```python
from build123d import *

# Parameters (mm, degrees)
SKETCH1_R           = 22.5
SKETCH1_R_2         = 20
BOSS_EXTRUDE1_DEPTH = 3
SKETCH2_R           = 1.25
BOSS_EXTRUDE2_DEPTH = 3
CIRPATTERN1_COUNT   = 2
SKETCH3_R           = 6.6
BOSS_EXTRUDE3_DEPTH = 3
SKETCH4_R           = 2
CUT_EXTRUDE1_DEPTH  = 3


with BuildPart() as part:
    # Sketch1 → Boss-Extrude1 (new body)
    with BuildSketch(Plane(origin=(0, 0, 0), x_dir=(1, 0, 0), z_dir=(0, 1, 0))):
        with Locations(Location((0, 0, 0), (0, 0, 270))):
            Circle(SKETCH1_R)
        with Locations(Location((0, 0, 0), (0, 0, 270))):
            Circle(SKETCH1_R_2, mode=Mode.SUBTRACT)
    extrude(amount=BOSS_EXTRUDE1_DEPTH)

    # Sketch2 → Boss-Extrude2 (add)
    with BuildSketch(Plane(origin=(0, 0, 0), x_dir=(1, 0, 0), z_dir=(0, 1, 0))):
        with BuildLine():
            Line((-2.5, 27), (2.5, 27))
            Line((2.5, 27), (2.5, 22.360679775))
            ThreePointArc((2.5, 22.360679775), (0, 22.5), (-2.5, 22.360679775))
            Line((-2.5, 22.360679775), (-2.5, 27))
        make_face()
        with Locations(Location((0, 24.7, 0), (0, 0, 270))):
            Circle(SKETCH2_R, mode=Mode.SUBTRACT)
    boss_extrude2 = extrude(amount=BOSS_EXTRUDE2_DEPTH)

    # CirPattern1: Boss-Extrude2 ×2 about axis
    cirpattern1_axis = Axis((0, 0, 0), (0, 1, 0))
    for i in range(1, CIRPATTERN1_COUNT):
        add(boss_extrude2.rotate(cirpattern1_axis, i * 360 / CIRPATTERN1_COUNT))

    # Sketch3 → Boss-Extrude3 (add)
    with BuildSketch(Plane(origin=(0, 0, 0), x_dir=(1, 0, 0), z_dir=(0, 1, 0))):
        with BuildLine():
            Line((-3, 19.773719933), (-3, 7.95298686))
            ThreePointArc((-3, 7.95298686), (-6.535301084, 5.435056554), (-8.366600265, 1.5))
            Line((-8.366600265, 1.5), (-19.943670675, 1.5))
            ThreePointArc((-19.943670675, 1.5), (-20, 0), (-19.943670675, -1.5))
            Line((-19.943670675, -1.5), (-8.366600265, -1.5))
            ThreePointArc((-8.366600265, -1.5), (-6.535301084, -5.435056554), (-3, -7.95298686))
            Line((-3, -7.95298686), (-3, -19.773719933))
            ThreePointArc((-3, -19.773719933), (0, -20), (3, -19.773719933))
            Line((3, -19.773719933), (3, -7.95298686))
            ThreePointArc((3, -7.95298686), (6.535301084, -5.435056554), (8.366600265, -1.5))
            Line((8.366600265, -1.5), (19.943670675, -1.5))
            ThreePointArc((19.943670675, -1.5), (20, 0), (19.943670675, 1.5))
            Line((19.943670675, 1.5), (8.366600265, 1.5))
            ThreePointArc((8.366600265, 1.5), (6.535301084, 5.435056554), (3, 7.95298686))
            Line((3, 7.95298686), (3, 19.773719933))
            ThreePointArc((3, 19.773719933), (0, 20), (-3, 19.773719933))
        make_face()
        with Locations(Location((0, 0, 0), (0, 0, 270))):
            Circle(SKETCH3_R, mode=Mode.SUBTRACT)
    extrude(amount=BOSS_EXTRUDE3_DEPTH)

    # Sketch4 → Cut-Extrude1 (cut)
    with BuildSketch(Plane(origin=(0, 3, 0), x_dir=(1, 0, 0), z_dir=(0, 1, 0))):
        with Locations(Location((0, 12.5, 0), (0, 0, 270))):
            Circle(SKETCH4_R)
        with Locations(Location((0, -12.5, 0), (0, 0, 270))):
            Circle(SKETCH4_R)
    extrude(amount=-CUT_EXTRUDE1_DEPTH, mode=Mode.SUBTRACT)


solid = part.part
```
Can you work these out from the model? Positions are in its coordinate system, mm. A direction names the side the tool comes from. Coordinates: 2 decimals unless noted, no trailing zeros. Order: outer loops, then holes, each group sorted by start corner. A loop starts at its lowest first (then second) coordinate and runs counter-clockwise, first axis right, second up. Notation, with made-up numbers: (35, 35.5) - (43, 35.5) arc R15 cw to (43, 60.5) - close; hole circle Ø2 at (20, -8). An arc over 180 degrees is marked (long way). Answer in a Markdown table with one row per item.
1. If we mould it in two halves opening along Z, with no side actions, what happens to faces 5 (the cylindrical face through (-14.537, 1.479, -13.736)), 6 (the flat face through (-3.4, 0, 5.9)), 7 (the flat face through (0, 1, 27)), 8 (the flat face through (-3, 1, 14))? For each: pulls with the +Z half, pulls with the -Z half, needs draft (parallel to the pull), parting line crosses it, or undercut.
Reply:
| item | result |
|---|---|
| face 5 | undercut |
| face 6 | needs draft |
| face 7 | pulls with the +Z half |
| face 8 | undercut |
2. Suppose I cut it at A-A (z = -24.7). Please give me the cut outline in (x, y).
Reply:
| item | result |
|---|---|
| outline | (-2.5, 0) - (-1.25, 0) - (-1.25, 3) - (-2.5, 3) - close; (1.25, 0) - (2.5, 0) - (2.5, 3) - (1.25, 3) - close |
3. For faces 1 (the flat face through (-2.5, 1, -25)), 2 (the flat face through (2.5, 1, -25)), 3 (the flat face through (-2.5, 1, 25)), 4 (the cylindrical face through (6.5, 1.48, 5.48)), which set-ups out of +Z, -Z, +X, -X, +Y, -Y let a thin tool reach every point of the face, with its end or its side?
Reply:
| item | result |
|---|---|
| face 1 | -Z, -X, +Y, -Y |
| face 2 | -Z, +X, +Y, -Y |
| face 3 | +Z, -X, +Y, -Y |
| face 4 | +Y, -Y |
4. If I drill on line 1 along X through (y, z) = (1, -17); line 2 along Z through (x, y) = (8.5, 1.25); line 3 along X through (y, z) = (2.95, -12), over which ranges is the centre line in solid material (lowest first)?
Reply:
| item | result |
|---|---|
| line 1 | x = -14.74 to -10.54, -3 to 3, 10.54 to 14.74 |
| line 2 | z = -20.83 to -18.1, -1.5 to 1.5, 18.1 to 20.83 |
| line 3 | x = -19.03 to -16, -3 to -1.94, 1.94 to 3, 16 to 19.03 |
5. Suppose I cut it at B-B (x = 0). Please give me the cut outline in (y, z).
Reply:
| item | result |
|---|---|
| outline | (0, -27) - (3, -27) - (3, -25.95) - (0, -25.95) - close; (0, -23.45) - (3, -23.45) - (3, -14.5) - (0, -14.5) - close; (0, -10.5) - (3, -10.5) - (3, -6.6) - (0, -6.6) - close; (0, 6.6) - (3, 6.6) - (3, 10.5) - (0, 10.5) - close; (0, 14.5) - (3, 14.5) - (3, 23.45) - (0, 23.45) - close; (0, 25.95) - (3, 25.95) - (3, 27) - (0, 27) - close |
6. Suppose I cut it at C-C (y = 0.9). Give the number of separate pieces and of enclosed holes in the cut face, and give its area (3 significant figures).
Reply:
| item | result |
|---|---|
| separate pieces | 1 |
| enclosed holes | 9 |
| area | 643 mm^2 |
7. Suppose I cut it at D-D (z = -12.5). Please give me the cut outline in (x, y), and give its area (3 significant figures).
Reply:
| item | result |
|---|---|
| outline | (-18.71, 0) - (-15.61, 0) - (-15.61, 3) - (-18.71, 3) - close; (-3, 0) - (-2, 0) - (-2, 3) - (-3, 3) - close; (2, 0) - (3, 0) - (3, 3) - (2, 3) - close; (15.61, 0) - (18.71, 0) - (18.71, 3) - (15.61, 3) - close |
| area | 24.6 mm^2 |
8. For pin 1 (0.9 mm diameter, centred on x = 16.5, y = 2, fed in from -Z); pin 2 (0.9 mm diameter, centred on y = 2, z = -13.5, fed in from +X); pin 3 (1.5 mm diameter, centred on y = 1, z = -12, fed in from -X); pin 4 (2 mm diameter, centred on x = 0, z = 24.7, fed in from -Y), each with a flat end and sliding along its axis, tell me the tip position at first contact or that it passes through.
Reply:
| item | result |
|---|---|
| pin 1 | stops at z = -15.77 |
| pin 2 | stops at x = 18.33 |
| pin 3 | stops at x = -19.49 |
| pin 4 | passes through |
